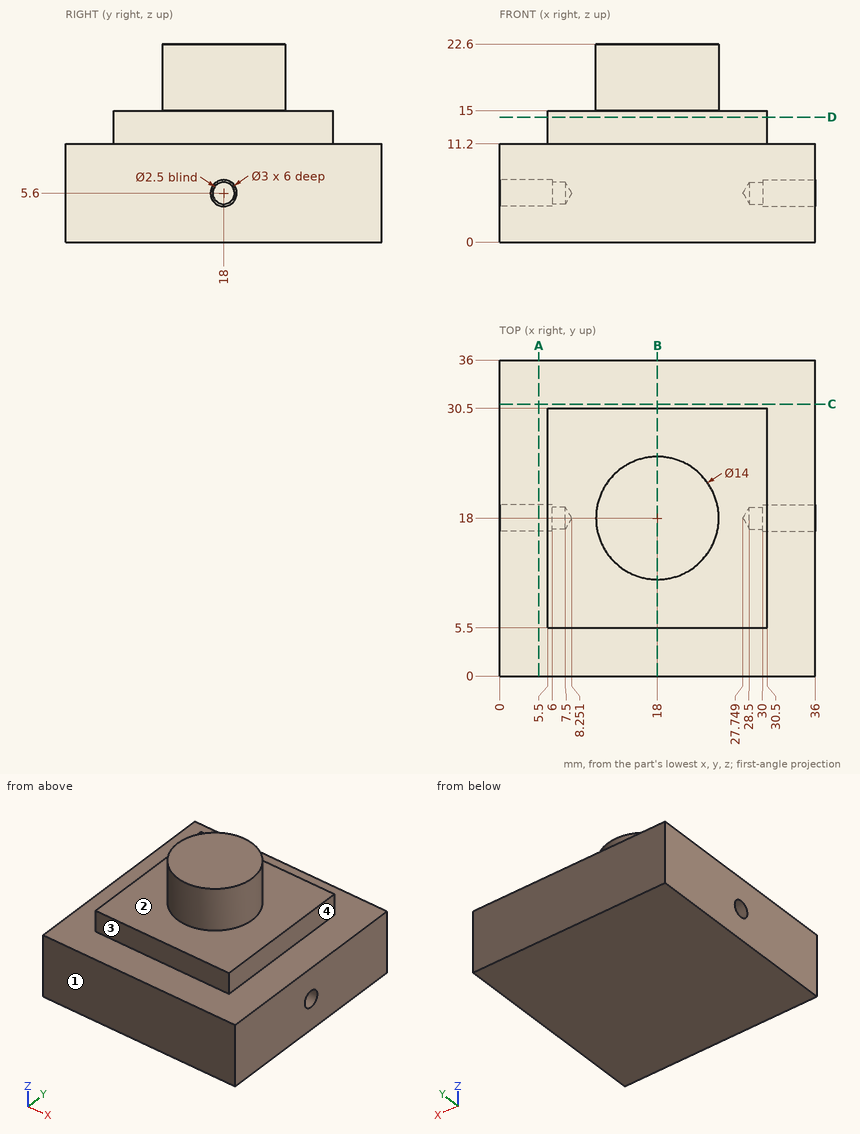
Verification items for this drawing (mm, ordinates from the low corner). A direction names the side the tool comes from. Give positions to 0.01 mm unless a question says otherwise; leave off trailing zeros. Write each loop counter-clockwise with the first axis right and the second up, starting at its lowest first coordinate (ties: lowest second). Pieces come first, ordered by that corner, then holes. Notation, with made-up numbers: (-20.5, 6) - (15.5, 6) arc R14 ccw to (15.5, 32) - close; hole circle Ø1 at (18.25, 7). An arc over 180 degrees is marked (long way). Answer as a JSON object with one key per item and string values. Group by question number.
1) Access from +Z, -Z, +X, -X, +Y, -Y to the whole of each face (thin tool, end or side, straight path). Record for the marked faces 1, 2, 3 and 4.
2) Sectioned sample at D-D (z = 14.25). Record the cut outline in (x, y), then the cut area to 3 significant figures.
3) Thickness scan on probe 1 along Y at (x, z) = (7.05, 5.6); probe 2 along Z at (x, y) = (4.5, 18); probe 3 along Z at (x, y) = (10.5, 5). Record the ranges inside material, lowest first. Write a range as from..to.
4) Sectioned sample at C-C (y = 31). Record the cut outline in (x, z), then the cut area to 3 significant figures.
5) Sectioned sample at A-A (x = 4.5). Record the cut outline in (y, z).
6) Depth check by flat-ended pin: P1, Ø3, axis at y = 12, z = 13, coming from the -X side; P2, Ø10, axis at x = 19, z = 19.5, coming from the +Y side; P3, Ø2, axis at y = 18, z = 5.6, coming from the -X side; P4, Ø2, axis at x = 32, z = 13, coming from the +Y side. Enter the tip coordinate at first touch or a pass-through.
7) Sectioned sample at B-B (x = 18). Record the cut outline in (y, z), then the cut area to 3 significant figures.
Geometry results:
{
 "1": {"face 1": "+Z, -Z, +X, -X, -Y", "face 2": "+Z", "face 3": "+Z, +X, -X, -Y", "face 4": "+Z, +X, +Y, -Y"},
 "2": {"outline": "(5.5, 5.5) - (30.5, 5.5) - (30.5, 30.5) - (5.5, 30.5) - close", "area": "625 mm^2"},
 "3": {"probe 1": "y = 0..16.75, 19.25..36", "probe 2": "z = 0..4.1, 7.1..11.2", "probe 3": "z = 0..11.2"},
 "4": {"outline": "(0, 0) - (36, 0) - (36, 11.2) - (0, 11.2) - close", "area": "403 mm^2"},
 "5": {"outline": "(0, 0) - (36, 0) - (36, 11.2) - (0, 11.2) - close; hole circle Ø3 at (18, 5.6)"},
 "6": {"P1": "stops at x = 5.5", "P2": "stops at y = 30.5", "P3": "stops at x = 7.65", "P4": "passes through"},
 "7": {"outline": "(0, 0) - (36, 0) - (36, 11.2) - (30.5, 11.2) - (30.5, 15) - (25, 15) - (25, 22.6) - (11, 22.6) - (11, 15) - (5.5, 15) - (5.5, 11.2) - (0, 11.2) - close", "area": "605 mm^2"}
}
